from build123d import *

# Parameters (mm, degrees)
F0_W     = 23
F0_H     = 27
F1_DEPTH = 32.85
F2_W     = 17
F2_H     = 19.25
F3_DEPTH = 32.851
F5_DEPTH = 27.001
F7_D     = 3.25
F7_DEPTH = 8
F7_TIP   = 0.9763985059


# Not quite as in the source:
# - a feature names something its author has since deleted; it is built from what else it names


with BuildPart() as f1:
    # F0 (on Front) → F1 (new body)
    with BuildSketch(Plane.XZ):
        Rectangle(F0_W, F0_H)
    extrude(amount=F1_DEPTH)

    # F2 (on face) → F3 (cut, through all)
    with BuildSketch(Plane.XZ.offset(32.85)):
        with Locations((1, -1.675)):
            Rectangle(F2_W, F2_H)
    extrude(amount=-F3_DEPTH, mode=Mode.SUBTRACT)

    # F4 (on face) → F5 (cut, through all)
    with BuildSketch(Plane.XY.offset(13.5)):
        Polygon((-11.5, -22.35), (8.4, 0), (-11.5, 0), align=None)
    extrude(amount=-F5_DEPTH, mode=Mode.SUBTRACT)

    # F7
    with Locations(Plane(origin=(-11.5, 0, 0), x_dir=(0, -1, 0), z_dir=(-1, 0, 0))):
        with Locations((25.7, 7.4)):
            Hole(F7_D / 2, depth=F7_DEPTH)
            with Locations((0, 0, -(F7_DEPTH + F7_TIP / 2))):  # 118° drill point
                Cone(0, F7_D / 2, F7_TIP, mode=Mode.SUBTRACT)


solid = f1.part
Source: CAD feature listing. Evaluate the final solid. Frame: model axes, mm. A direction names the side the tool comes from. Coordinates: 2 decimals unless noted, no trailing zeros. Loops run counter-clockwise (first coordinate to the right, second up) from the corner with the lowest first, then second, coordinate; pieces in that order, holes last. Notation, with made-up numbers: (9, 56.25) - (15, 56.25) arc R26 ccw to (15, 89.25) - close; hole circle Ø7 at (14.25, -38.5). An arc over 180 degrees is marked (long way). One line per question, with ' | ' between items.
1) Section B-B, the plane y = -25.7. Return loops of the section in (x, z) (3 decimals), then the cut area to 3 significant figures.
Report:
outline: (-11.5, -13.5) - (11.5, -13.5) - (11.5, 13.5) - (-11.5, 13.5) - (-11.5, 9.025) - (-3.5, 9.025) - (-2.854, 7.95) - (9.5, 7.95) - (9.5, -11.3) - (-7.5, -11.3) - (-7.5, 5.775) - (-11.5, 5.775) - close | area: 276 mm²
2) Section D-D, the plane z = 1. Return loops of the section in (x, y).
Report:
outline: (-11.5, -32.85) - (-7.5, -32.85) - (-7.5, -17.86) - (-11.5, -22.35) - close; (9.5, -32.85) - (11.5, -32.85) - (11.5, 0) - (9.5, 0) - close
3) Line query: line 1 along Z through (x, y) = (7, -10); line 2 along Z through (x, y) = (-6.25, -25.7) (3 decimals); line 3 along X through (y, z) = (-31, -2.75). Output: solid intervals per line, ascending.
Report:
line 1: z = -13.5 to -11.3, 7.95 to 13.5 | line 2: z = -13.5 to -11.3, 9.025 to 13.5 | line 3: x = -11.5 to -7.5, 9.5 to 11.5
4) Pull-direction query (Z, two-part tool) for faces 4 (the face through (-3.107, -25.717, 8.371)), 5 (the face through (2, -20, 13.5)), 6 (the face through (10, 0, 0)), 7 (the face through (2, -20, -13.5)); classes: released by +Z, released by -Z, zero draft, split by the parting line, or undercut.
Report:
face 4: undercut | face 5: released by +Z | face 6: zero draft | face 7: released by -Z
5) Section A-A, the plane z = 7.4. Return loops of the section in (x, y) (3 decimals), then the cut area to 3 significant figures.
Report:
outline: (-11.5, -32.85) - (-7.5, -32.85) - (-7.5, -27.325) - (-11.5, -27.325) - close; (-11.5, -24.075) - (-7.5, -24.075) - (-7.5, -17.858) - (-11.5, -22.35) - close; (9.5, -32.85) - (11.5, -32.85) - (11.5, 0) - (9.5, 0) - close | area: 104 mm²
6) First-contact query: P1, Ø5, axis at x = -7.5, z = 1, coming from the +Y side; P2, Ø6, axis at y = -14, z = -0.5, coming from the -X side. Flat tips, straight axial feed; report the tip coordinate or a pass-through.
Report:
P1: stops at y = -17.86 | P2: stops at x = 9.5
7) Set-up query: faces 1 (the face through (-11.5, -28, 0)), 2 (the face through (3, -20, 7.95)), 3 (the face through (-8.33, -25.91, 9.01)). Return all of +Z, -Z, +X, -X, +Y, -Y with unobstructed straight access to the full face (end or side cutting, diameter ignored); none if empty.
Report:
face 1: +Z, -Z, -X, +Y, -Y | face 2: +Y, -Y | face 3: -X
8) Section C-C, the plane x = 6. Return loops of the section in (y, z), then the cut area to 3 significant figures.
Report:
outline: (-32.85, -13.5) - (-2.7, -13.5) - (-2.7, -11.3) - (-32.85, -11.3) - close; (-32.85, 7.95) - (-2.7, 7.95) - (-2.7, 13.5) - (-32.85, 13.5) - close | area: 234 mm²
